Design review of the part shown in the three views and the two pictorial views. Dimensions are in mm from the part's minimum x, y and z. A direction names the side the tool comes from. Round coordinates to 2 decimals unless told otherwise and drop trailing zeros. Write each loop counter-clockwise with the first axis right and the second up, starting at its lowest first coordinate (ties: lowest second). Pieces come first, ordered by that corner, then holes. Notation, with made-up numbers: (-28.5, -25) -> (13.5, -25) arc R16 cw to (13.5, 4) -> close; hole circle Ø2 at (8.25, 10.5). An arc over 180 degrees is marked (long way). Answer as a JSON object with one key per item and string values. Group by question number.
1) We need section A-A, the plane y = 36.5. Write out the cut boundary in (x, z) (1 decimal).
2) We need section C-C, the plane z = 4.7. Count the separate pieces of the cut face and the enclosed holes in it, then the cut area to 3 significant figures.
3) Insertion check: pin 1 Ø3 at (x, z) = (14, 3) entering from +Y; pin 2 Ø3 at (y, z) = (21, 3.5) entering from +X; pin 3 Ø2 at (y, z) = (56, 1.5) entering from -X; pin 4 Ø1 at (y, z) = (52, 2.5) entering from -X. Each pin has a flat end and moves straight along its axis. Give the tip position at first contact, or say it passes through.
4) We need section B-B, the plane x = 23.89. Write out the cut boundary in (y, z) (1 decimal), then the cut area to 3 significant figures.
5) Machinability: for the marked faces 4, 5 and 6, which of the approach directions +Z, -Z, +X, -X, +Y, -Y give a long, thin tool a straight path to every point of the face, cutting with its end or side? Answer none if there is none.
6) Mouldability with a two-part tool opening along Y and no side actions: class the marked faces 1, 2 and 3 as pulls with the +Y half, pulls with the -Y half, needs draft (parallel to the pull), parting line crosses it, or undercut.
7) We need section D-D, the plane x = 43. Write out the cut boundary in (y, z) (1 decimal).
8) To check wall thickness, follow probe 1 along Y at (x, z) = (23.89, 3.2); probe 2 along Y at (x, z) = (43, 3.3); probe 3 along X at (y, z) = (35, 4.3) (1 decimal). State the ranges of each line that lie inside material, in increasing order. Write a range as [from, to].
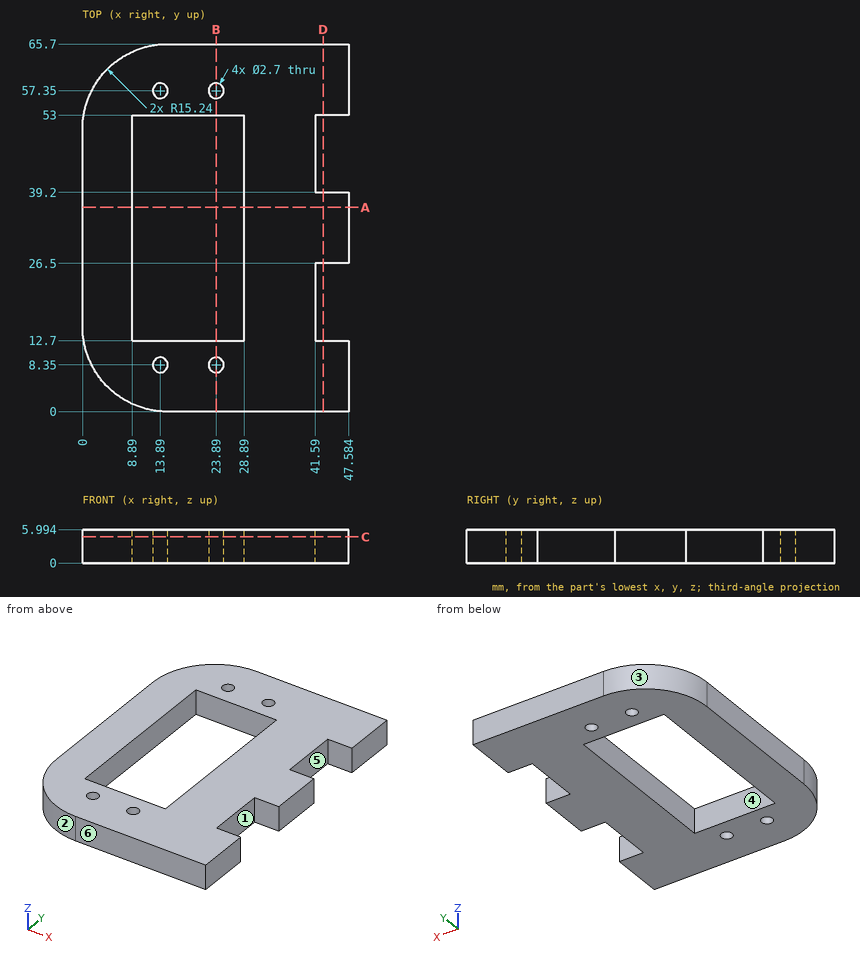
Here are the results:
{
 "1": {"outline": "(0, 0) -> (8.9, 0) -> (8.9, 6) -> (0, 6) -> close; (28.9, 0) -> (47.6, 0) -> (47.6, 6) -> (28.9, 6) -> close"},
 "2": {"separate pieces": "1", "enclosed holes": "5", "area": "2,030 mm^2"},
 "3": {"pin 1": "stops at y = 65.7", "pin 2": "stops at x = 41.59", "pin 3": "stops at x = 0.69", "pin 4": "stops at x = 0.04"},
 "4": {"outline": "(0, 0) -> (7, 0) -> (7, 6) -> (0, 6) -> close; (9.7, 0) -> (12.7, 0) -> (12.7, 6) -> (9.7, 6) -> close; (53, 0) -> (56, 0) -> (56, 6) -> (53, 6) -> close; (58.7, 0) -> (65.7, 0) -> (65.7, 6) -> (58.7, 6) -> close", "area": "120 mm^2"},
 "5": {"face 4": "+Z, -Z", "face 5": "+Z, -Z, +X", "face 6": "+Z, -Z, +X, -X, -Y"},
 "6": {"face 1": "undercut", "face 2": "pulls with the -Y half", "face 3": "pulls with the +Y half"},
 "7": {"outline": "(0, 0) -> (12.7, 0) -> (12.7, 6) -> (0, 6) -> close; (26.5, 0) -> (39.2, 0) -> (39.2, 6) -> (26.5, 6) -> close; (53, 0) -> (65.7, 0) -> (65.7, 6) -> (53, 6) -> close"},
 "8": {"probe 1": "y = [0, 7], [9.7, 12.7], [53, 56], [58.7, 65.7]", "probe 2": "y = [0, 12.7], [26.5, 39.2], [53, 65.7]", "probe 3": "x = [0, 8.9], [28.9, 47.6]"}
}
